from build123d import *

# Parameters (mm, degrees)
ESBO_O1_W                = 12
ESBO_O1_H                = 12
RESSALTO_EXTRUS_O1_DEPTH = 2
FILETE1_R                = 2


with BuildPart() as part:
    # Esboço1 → Ressalto-extrusão1 (new body)
    with BuildSketch(Plane.XY):
        Rectangle(ESBO_O1_W, ESBO_O1_H)
    extrude(amount=RESSALTO_EXTRUS_O1_DEPTH)

    # Filete1
    filete1_edges = [part.edges().sort_by_distance(p)[0] for p in [
        (-6, 6, 1),
        (6, 6, 1),
        (6, -6, 1),
        (-6, -6, 1),
    ]]
    fillet(filete1_edges, radius=FILETE1_R)


solid = part.part
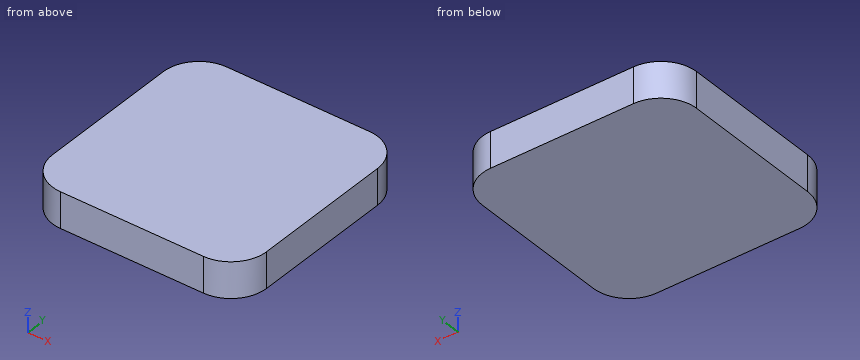
Input: part model. Units: mm. Frame: model coordinates. Coordinates: 2 decimals unless noted, no trailing zeros. Loops run counter-clockwise (first coordinate to the right, second up) from the corner with the lowest first, then second, coordinate; pieces in that order, holes last. Notation, with made-up numbers: (53.5, 62) - (61.5, 62) arc R8 ccw to (61.5, 70) - close; hole circle Ø2 at (-11.75, -9.5). An arc over 180 degrees is marked (long way). Answer in a Markdown table with one row per item. Add a question column.
Item 1: Line query: line 1 along Y through (x, z) = (5.25, 0.75); line 2 along Y through (x, z) = (4.5, 1.65). Output: solid intervals per line, ascending. Write a range as [from, to].
Item 2: Section query B-B on y = -5. Return the cut outline in (x, z), then the cut area to 3 significant figures.
Item 3: Section query A-A on z = 1.7. Return the cut outline in (x, y), then the cut area to 3 significant figures.
Recorded:
| question | item | result |
|---|---|---|
| 1 | line 1 | [-5.56, 5.56] |
| 1 | line 2 | [-5.94, 5.94] |
| 2 | outline | (-5.73, 0) - (5.73, 0) - (5.73, 2) - (-5.73, 2) - close |
| 2 | area | 22.9 mm^2 |
| 3 | outline | (-6, -4) arc R2 ccw to (-4, -6) - (4, -6) arc R2 ccw to (6, -4) - (6, 4) arc R2 ccw to (4, 6) - (-4, 6) arc R2 ccw to (-6, 4) - close |
| 3 | area | 141 mm^2 |
